Model file for the job. Use its own axes, mm. Give positions to 0.01 mm unless a question says otherwise; leave off trailing zeros. Order: outer loops, then holes, each group sorted by start corner. A loop starts at its lowest first (then second) coordinate and runs counter-clockwise, first axis right, second up. Notation, with made-up numbers: (19, 76.5) -> (71, 76.5) arc R8 cw to (71, 86.5) -> close; hole circle Ø6 at (-32, 32.5). An arc over 180 degrees is marked (long way). Answer in a Markdown table with one row per item. Add a question column.
from build123d import *

# Parameters (mm, degrees)
ESBO_O1_W                = 555
ESBO_O1_H                = 200
RESSALTO_EXTRUS_O1_DEPTH = 3
ESBO_O2_W                = 3.5
ESBO_O2_H                = 31
ESBO_O2_W_2              = 31
ESBO_O2_H_2              = 3.5
CORTE_EXTRUS_O1_DEPTH    = 295.983474113
ESBO_O3_OUTSIDE_W        = 674.988
ESBO_O3_OUTSIDE_H        = 319.988
CORTE_EXTRUS_O3_DEPTH    = 295.983474113


with BuildPart() as part:
    # Esboço1 → Ressalto-extrusão1 (new body)
    with BuildSketch(Plane.XY):
        Rectangle(ESBO_O1_W, ESBO_O1_H)
    extrude(amount=RESSALTO_EXTRUS_O1_DEPTH)

    # Esboço2 → Corte-extrusão1 (cut, through all)
    with BuildSketch(Plane.XY.offset(3)):
        with Locations((237.25, 0)):
            Rectangle(ESBO_O2_W, ESBO_O2_H)
        with Locations((-153.75, 0)):
            Rectangle(ESBO_O2_W, ESBO_O2_H)
        with Locations((-237.25, 0)):
            Rectangle(ESBO_O2_W, ESBO_O2_H)
        with Locations((-195.5, 41.75)):
            Rectangle(ESBO_O2_W_2, ESBO_O2_H_2)
        with Locations((-195.5, -41.75)):
            Rectangle(ESBO_O2_W_2, ESBO_O2_H_2)
        with Locations((153.75, 0)):
            Rectangle(ESBO_O2_W, ESBO_O2_H)
        with Locations((195.5, -41.75)):
            Rectangle(ESBO_O2_W_2, ESBO_O2_H_2)
        with Locations((195.5, 41.75)):
            Rectangle(ESBO_O2_W_2, ESBO_O2_H_2)
    extrude(amount=-CORTE_EXTRUS_O1_DEPTH, mode=Mode.SUBTRACT)

    # Esboço3 outside → Corte-extrusão3 (cut, through all)
    with BuildSketch(Plane.XY.offset(3)):
        Rectangle(ESBO_O3_OUTSIDE_W, ESBO_O3_OUTSIDE_H)
        Polygon((0, 100), (0, 50), (15, 50), (15, -50), (0, -50), (0, -100), (277.5, -100), (277.5, 100), align=None, mode=Mode.SUBTRACT)
    extrude(amount=-CORTE_EXTRUS_O3_DEPTH, mode=Mode.SUBTRACT)


solid = part.part
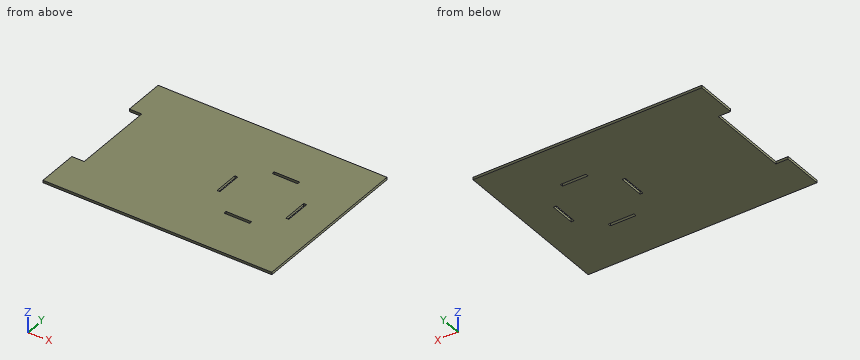
Item 1: Saw through at D-D on y = -24. List the corners of the cut face in (x, z).
Item 2: Saw through at A-A on y = 1. List the corners of the cut face in (x, z), plus the area to 4 significant figures.
Item 3: Wall check: line 1 (X direction, y = 3.5, z = 2.85); line 2 (Y direction, x = 182, z = 1.1); line 3 (Y direction, x = 237.5, z = 2.25). Give the ranges that are in metal, low to high.
Item 4: Pin check, flat tips, straight feed: pin 1 Ø2 at (x, y) = (135, 43) entering from -Z; pin 2 Ø0.9 at (y, z) = (6, 1.5) entering from -X. Stop position of each tip, or through.
Item 5: Saw through at B-B on x = 208. List the corners of the cut face in (y, z).
Item 6: Saw through at C-C on z = 2.35. List the corners of the cut face in (x, y), plus the area to 3 significant figures.
Evaluation:
| question | item | result |
|---|---|---|
| 1 | outline | (15, 0) -> (277.5, 0) -> (277.5, 3) -> (15, 3) -> close |
| 2 | outline | (15, 0) -> (152, 0) -> (152, 3) -> (15, 3) -> close; (155.5, 0) -> (235.5, 0) -> (235.5, 3) -> (155.5, 3) -> close; (239, 0) -> (277.5, 0) -> (277.5, 3) -> (239, 3) -> close |
| 2 | area | 766.5 mm2 |
| 3 | line 1 | x = 15 to 152, 155.5 to 235.5, 239 to 277.5 |
| 3 | line 2 | y = -100 to -43.5, -40 to 40, 43.5 to 100 |
| 3 | line 3 | y = -100 to -15.5, 15.5 to 100 |
| 4 | pin 1 | stops at z = 0 |
| 4 | pin 2 | stops at x = 15 |
| 5 | outline | (-100, 0) -> (-43.5, 0) -> (-43.5, 3) -> (-100, 3) -> close; (-40, 0) -> (40, 0) -> (40, 3) -> (-40, 3) -> close; (43.5, 0) -> (100, 0) -> (100, 3) -> (43.5, 3) -> close |
| 6 | outline | (0, -100) -> (277.5, -100) -> (277.5, 100) -> (0, 100) -> (0, 50) -> (15, 50) -> (15, -50) -> (0, -50) -> close; hole (152, -15.5) -> (155.5, -15.5) -> (155.5, 15.5) -> (152, 15.5) -> close; hole (180, -43.5) -> (211, -43.5) -> (211, -40) -> (180, -40) -> close; hole (180, 40) -> (211, 40) -> (211, 43.5) -> (180, 43.5) -> close; hole (235.5, -15.5) -> (239, -15.5) -> (239, 15.5) -> (235.5, 15.5) -> close |
| 6 | area | 53,600 mm2 |
